Check sheet for the modelled part. Datum: model origin and axes. Units: mm. A direction names the side the tool comes from. Round coordinates to 2 decimals unless told otherwise and drop trailing zeros. Order: outer loops, then holes, each group sorted by start corner. A loop starts at its lowest first (then second) coordinate and runs counter-clockwise, first axis right, second up. Notation, with made-up numbers: (54, 39.5) -> (64, 39.5) arc R21 ccw to (64, 72.5) -> close; hole circle Ø3 at (76.5, -11). An arc over 180 degrees is marked (long way). Answer in a Markdown table with one row per item. Add a question column.
1. Material ranges on L1, parallel to X at y = -25, z = 1.7; L2, parallel to X at y = -0.5, z = 1.5; L3, parallel to Y at x = -47, z = 2.25, recorded low to high. Write a range as from..to.
2. Draft check along Y on faces 1 (the flat face through (-1, 32.5, 2)), 2 (the flat face through (-38, -26.5, 2)), 3 (the flat face through (-5, -33, 2)). Enter one of: +Y half, -Y half, draft (parallel to the pull), parting line (faces both ways), or undercut.
3. Sectioned sample at B-B, the plane x = -45. Record the boundary of the cut face in (y, z).
4. Depth check by flat-ended pin: P1, Ø1.2, axis at y = -35.5, z = 1.5, coming from the +X side; P2, Ø1, axis at x = -17.5, z = 2, coming from the -Y side; P3, Ø2, axis at y = 15, z = 2, coming from the +X side. Enter the tip coordinate at first touch or a pass-through.
5. Access from +Z, -Z, +X, -X, +Y, -Y to the whole of each face (thin tool, end or side, straight path). Record for faces 4 (the flat face through (37, -26.5, 2)), 5 (the flat face through (0, -39.566, 2)).
6. Sectioned sample at A-A, the plane z = 2.65. Record the boundary of the cut face in (x, y).
```python
from build123d import *

# Parameters (mm, degrees)
BOSS_EXTRUDE1_DEPTH     = 4
SKETCH1_W               = 140
SKETCH1_H               = 53
BOSS_EXTRUDE2_DEPTH     = 4
BOSS_EXTRUDE3_DEPTH     = 4
CUT_EXTRUDE1_DEPTH      = 5
CUT_EXTRUDE1_DEPTH_BACK = 2
CUT_EXTRUDE4_DEPTH      = 81.533747288
CUT_EXTRUDE4_DEPTH_BACK = 81.533747288
SKETCH4_R               = 1


with BuildPart() as part:
    # Sketch3 → Boss-Extrude1 (new body)
    with BuildSketch(Plane.XY):
        Polygon((0, -26.5), (5, -26.5), (5, -39.566040215), (-4.99956385, -39.566040215), (-4.99956385, -26.566040215), (-4.99956385, -26.5), align=None)
    extrude(amount=BOSS_EXTRUDE1_DEPTH)

    # Sketch1 → Boss-Extrude2 (add)
    with BuildSketch(Plane.XY):
        Rectangle(SKETCH1_W, SKETCH1_H)
    extrude(amount=BOSS_EXTRUDE2_DEPTH)

    # Sketch5 → Boss-Extrude3 (add)
    with BuildSketch(Plane.XY):
        Polygon((-70, 26.5), (-70, 32.5), (70.030085777, 32.5), (70, 26.5), align=None)
    extrude(amount=BOSS_EXTRUDE3_DEPTH)

    # Sketch6 → Cut-Extrude1 (cut, two sides: drawn at the far end of the back side and taken through both)
    with BuildSketch(Plane.XY.offset(-CUT_EXTRUDE1_DEPTH_BACK)):
        with BuildLine():
            ThreePointArc((-67.496184759, 31), (-68.114088128, 31.924122375), (-69.204189088, 31.706208093))
            Line((-69.204189088, 31.706208093), (-67.78818043, 30.293791907))
            ThreePointArc((-67.78818043, 30.293791907), (-67.572062384, 30.617903369), (-67.496184759, 31))
        make_face()
        with BuildLine():
            Line((-67.78818043, 30.293791907), (-69.204189088, 31.706208093))
            ThreePointArc((-69.204189088, 31.706208093), (-69.202392852, 30.291995671), (-67.78818043, 30.293791907))
        make_face()
    extrude(amount=CUT_EXTRUDE1_DEPTH + CUT_EXTRUDE1_DEPTH_BACK, mode=Mode.SUBTRACT)

    # Sketch4 → Cut-Extrude4 (cut, two sides: drawn at the far end of the back side and taken through both)
    with BuildSketch(Plane.XY.offset(-CUT_EXTRUDE4_DEPTH_BACK)):
        with Locations((-68.496184759, -25)):
            Circle(SKETCH4_R)
        with Locations((68.503815241, -25)):
            Circle(SKETCH4_R)
        with Locations((68.518858129, 31)):
            Circle(SKETCH4_R)
    extrude(amount=CUT_EXTRUDE4_DEPTH + CUT_EXTRUDE4_DEPTH_BACK, mode=Mode.SUBTRACT)


solid = part.part
```
Answer key:
| question | item | result |
|---|---|---|
| 1 | L1 | x = -70..-69.5, -67.5..67.5, 69.5..70 |
| 1 | L2 | x = -70..70 |
| 1 | L3 | y = -26.5..32.5 |
| 2 | face 1 | +Y half |
| 2 | face 2 | -Y half |
| 2 | face 3 | draft |
| 3 | outline | (-26.5, 0) -> (32.5, 0) -> (32.5, 4) -> (-26.5, 4) -> close |
| 4 | P1 | stops at x = 5 |
| 4 | P2 | stops at y = -26.5 |
| 4 | P3 | stops at x = 70 |
| 5 | face 4 | +Z, -Z, +X, -Y |
| 5 | face 5 | +Z, -Z, +X, -X, -Y |
| 6 | outline | (-70, -26.5) -> (-5, -26.5) -> (-5, -39.57) -> (5, -39.57) -> (5, -26.5) -> (70, -26.5) -> (70, 26.5) -> (70.03, 32.5) -> (-70, 32.5) -> close; hole circle Ø2 at (-68.5, -25); hole circle Ø2 at (-68.5, 31); hole circle Ø2 at (68.5, -25); hole circle Ø2 at (68.52, 31) |
